Could you check a few things on this model? Use its own coordinates, in mm. Face numbers are marked on the shaded views. A direction names the side the tool comes from. Give positions to 0.01 mm unless a question says otherwise; leave off trailing zeros. Loops run counter-clockwise (first coordinate to the right, second up) from the corner with the lowest first, then second, coordinate; pieces in that order, holes last. Notation, with made-up numbers: M 49,23.5 L 82,23.5 A14 ccw 82,32.5 Z; hole C -34.75,-26 d5. An arc over 180 degrees is marked long. Use a Markdown table: item, result. Add a question column.
1) Which directions (+Z, -Z, +X, -X, +Y, -Y) give clear straight access to the entire face, cutting with the end or side of a thin tool? Please do the marked faces 1, 2 and 3.
2) Suppose I cut it at C-C on z = -62.75. List the corners of the cut face in (x, y) for me, and give its area (3 significant figures).
3) Suppose I cut it at B-B on y = 128.5. List the corners of the cut face in (x, z) for me, and give its area (3 significant figures).
4) Suppose I cut it at A-A on x = 18.8. List the corners of the cut face in (y, z) for me.
5) Will these pins go through, and if not, where does the flat tip stop? pin 1 Ø2 at (x, y) = (21, 142) entering from -Z; pin 2 Ø3 at (x, z) = (21, -53.5) entering from -Y; pin 3 Ø12 at (y, z) = (125, -51) entering from +X; pin 4 Ø3 at (x, z) = (18, -52) entering from +Y.
6) If I drill on line 1 along Z through (x, y) = (19.45, 132); line 2 along Y through (x, z) = (19.9, -56.25); line 3 along Z through (x, y) = (18, 150), over which ranges is the centre line in solid material (lowest first)? Write a range as [from, to].
Autodesk Inventor part; units mm, degrees
ref_plane "YZ Plane" through (0, 0, 0) normal (1, 0, 0) x (0, 1, 0)
ref_plane "XZ Plane" through (0, 0, 0) normal (0, 1, 0) x (-1, 0, 0)
ref_plane "XY Plane" through (0, 0, 0) normal (0, 0, 1) x (1, 0, 0)
ref_plane "Work Plane1" through (15.2715, 198.3363, -46.0983) normal (-1, 0, 0) x (0, 1, 0)
sketch "Sketch1" plane through (15.2715, 198.3363, -46.0983) normal (-1, 0, 0) x (0, 1, 0)
  line L0 (-57.2075, -5.2313) -> (-57.2075, -7.2313)
  line L1 (-59.3325, 28.2487) -> (-59.3325, 9.0387)
  line L2 (-39.0825, 28.2487) -> (-39.0825, 9.0387)
  line L3 (-60.777, -7.2313) -> (-38.43, -7.2313)
  line L4 (-38.43, -0.2313) -> (-60.777, -0.2313)
  line L5 (-113.6123, 22.7696) -> (-98.1523, 22.7696)
  line L6 (-105.2077, 22.7696) -> (-105.2077, -2.2304)
  line L7 (-105.2077, -2.2304) -> (-42.2077, -2.2304)
  point P0 (-198.3363, -46.0983)
  dimension "d0" = 25
  dimension "d1" = 63
ref_plane "Work Plane2" through (20.8129, 75.0546, -60.4371) normal (0, 0, -1) x (-1, 0, 0)
sketch "Sketch2" plane through (20.8129, 75.0546, -60.4371) normal (0, 0, -1) x (-1, 0, 0)
  circle A0 centre (0.9353, 17.3993) radius 7.73
  circle A1 centre (0.9353, 17.3993) radius 2.641
  point P0 (20.8129, -75.0546)
sweep "Sweep1" add profiles "Sketch2" path "Sketch1" path curves L6 L7 contours A1
sketch "Sketch3" plane through (15.2715, 198.3363, -46.0983) normal (-1, 0, 0) x (0, 1, 0)
  line L0 (-42.2077, -5.5462) -> (-42.2077, -0.2641)
  line L1 (-105.8823, -2.9051) -> (-105.8823, -2.9051)
  line L2 (-105.8823, -2.9051) -> (-105.8823, -2.9051)
  line L3 (-108.5234, 22.7696) -> (-103.2413, 22.7696)
  line L4 (-113.9183, 5.1309) -> (-96.4131, -12.3743)
  line L5 (-96.4131, -12.3743) -> (-115.0261, -30.9873)
  line L6 (-115.0261, -30.9873) -> (-132.5313, -13.4821)
  line L7 (-132.5313, -13.4821) -> (-113.9183, 5.1309)
  line L8 (-113.9183, 5.1309) -> (-89.1622, 5.1309) construction
  line L9 (-105.8823, 22.7696) -> (-105.8823, -27.9051)
  line L10 (-105.8823, -2.9051) -> (-105.8823, -2.9051)
  line L11 (-105.8823, -2.9051) -> (-105.8823, -2.9051)
  point P0 (-198.3363, -46.0983)
  dimension "d4" = 45
extrude "Extrusion1" cut sketch "Sketch3" along normal mid plane 10
sketch "Sketch4" plane through (19.8776, 92.454, -43.1932) normal (0, -0.7071, 0.7071) x (1, 0, 0)
  ellipse E0 centre (0, 0) end of major axis (0, -3.735) minor radius 2.641 (0.3939, 3.6932) -> (-2.641, 0) ccw
  ellipse E1 centre (0, 0) end of major axis (0, 3.735) minor radius 2.641 (-2.641, 0) -> (0.3939, -3.6932) ccw
  circle A0 centre (0, 0) radius 1.9322
  point P0 (-19.8776, -34.8326)
  point P1 (2.641, 0)
extrude "Extrusion2" cut sketch "Sketch4" against normal blind 10
properties part number "00_opticalpath"
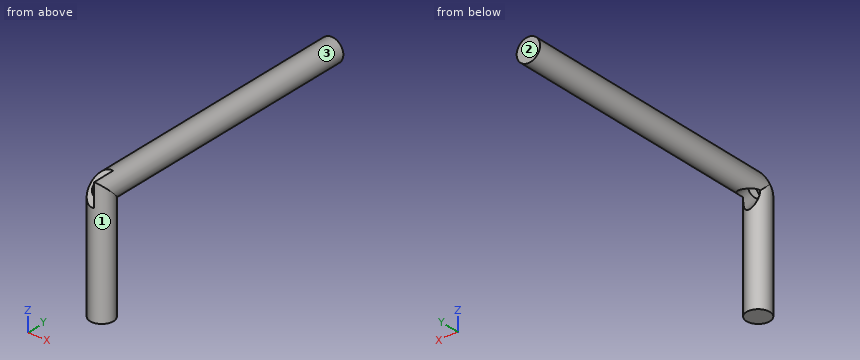
Answer block:
| question | item | result |
|---|---|---|
| 1 | face 1 | -Z |
| 1 | face 2 | +Z, -Z, +X, -X, +Y |
| 1 | face 3 | +Y |
| 2 | outline | C 19.88,92.45 d5.28 |
| 2 | area | 21.9 mm^2 |
| 3 | outline | C 19.88,-43.19 d5.28 |
| 3 | area | 21.9 mm^2 |
| 4 | outline | M 90.04,-68.87 L 94.87,-68.87 L 94.87,-47.87 L 91.32,-44.33 L 90.04,-45.6 Z; M 93.59,-42.06 L 97.13,-45.6 L 156.13,-45.6 L 156.13,-40.78 L 94.87,-40.78 Z |
| 5 | pin 1 | stops at z = -45.83 |
| 5 | pin 2 | stops at y = 89.81 |
| 5 | pin 3 | stops at x = 21.8 |
| 5 | pin 4 | stops at y = 95.07 |
| 6 | line 1 | z = [-45.8, -40.59] |
| 6 | line 2 | y = [89.81, 95.09] |
| 6 | line 3 | z = [-45.05, -41.34] |
